Input: part model. Units: mm. Frame: model coordinates. A direction names the side the tool comes from. Coordinates: 2 decimals unless noted, no trailing zeros. Write each loop counter-clockwise with the first axis right and the second up, starting at its lowest first coordinate (ties: lowest second). Pieces come first, ordered by that corner, then holes. Notation, with made-up numbers: (0, 46.25) -> (11, 46.25) arc R21 cw to (11, 82.25) -> close; hole circle Ø3 at (58.25, 12). An arc over 180 degrees is marked (long way). Use one line per item in the form item = value. Start each with the question number.
(1) Cut plane D-D on x = -10.5. Return the cut outline in (y, z), plus the area to 3 significant figures.
(2) Cut plane C-C on y = -8. Return the cut outline in (x, z).
(3) Ray query, line 1 along Y through (x, z) = (0, -14); line 2 along Y through (x, z) = (0, 155); line 3 along X through (y, z) = (0, -15.25). Return the intervals inside material, ascending.
(4) Set-up query: faces 1 (the face through (0, 0, 8.44)), 2 (the face through (-4, -4, -35)). Return all of +Z, -Z, +X, -X, +Y, -Y with unobstructed straight access to the full face (end or side cutting, diameter ignored); none if empty.
(5) First-contact query: pin 1 (1 mm diameter, centred on x = 14, y = 0.5, fed in from +Z); pin 2 (8 mm diameter, centred on x = -7.5, z = 121, fed in from +Y); pin 3 (5 mm diameter, centred on x = -1.5, z = 101.5, fed in from -Y); pin 4 (1.7 mm diameter, centred on x = 4.5, y = 0, fed in from -Z). Flat tips, straight axial feed; report the tip coordinate or a pass-through.
(6) Cut plane B-B on z = 141. Return the cut outline in (x, y).
(7) Cut plane A-A on x = 0. Return the cut outline in (y, z).
(8) Pull-direction query (X, two-part tool) for faces 3 (the face through (3, 15, 208.44)), 4 (the face through (-1, 0, -10)); classes: released by +X, released by -X, zero draft, split by the parting line, or undercut.
```python
from build123d import *

# Parameters (mm, degrees)
SKETCH_1_R          = 20
EXTRUDE_1_DEPTH     = 208.44
EXTRUDE_START       = 35
SKETCH_3_R          = 20
EXTRUDE_2_DEPTH     = 35
CUT_EXTRUDE_1_DEPTH = 25
SKETCH_5_R          = 5
CUT_EXTRUDE_2_DEPTH = 10
SKETCH_6_R          = 15
CUT_EXTRUDE_3_DEPTH = 200


with BuildPart() as part:
    # 스케치1 → 보스-돌출1 (new body)
    with BuildSketch(Plane.XY):
        Circle(SKETCH_1_R)
    extrude(amount=EXTRUDE_1_DEPTH)

    # 스케치3 → 보스-돌출2 (add)
    with BuildSketch(Plane(origin=(0, 0, 0), x_dir=(-1, 0, 0), z_dir=(0, 0, -1)).offset(EXTRUDE_START)):
        Circle(SKETCH_3_R)
    extrude(amount=-EXTRUDE_2_DEPTH)

    # 스케치4 → 컷-돌출1 (cut)
    with BuildSketch(Plane(origin=(0, 0, -35), x_dir=(-1, 0, 0), z_dir=(0, 0, -1))):
        with BuildLine():
            Line((-3.515670801, 3.555286039), (-3.484261495, -3.586073317))
            ThreePointArc((-3.484261495, -3.586073317), (4.99995164, 0.021990913), (-3.515670801, 3.555286039))
        make_face()
    extrude(amount=-CUT_EXTRUDE_1_DEPTH, mode=Mode.SUBTRACT)

    # 스케치5 → 컷-돌출2 (cut)
    with BuildSketch(Plane(origin=(0, 0, -35), x_dir=(-1, 0, 0), z_dir=(0, 0, -1))):
        Circle(SKETCH_5_R)
    extrude(amount=-CUT_EXTRUDE_2_DEPTH, mode=Mode.SUBTRACT)

    # 스케치6 → 컷-돌출3 (cut)
    with BuildSketch(Plane.XY.offset(208.44)):
        Circle(SKETCH_6_R)
    extrude(amount=-CUT_EXTRUDE_3_DEPTH, mode=Mode.SUBTRACT)


solid = part.part
```
Values:
q1.outline = (-17.02, -35) -> (17.02, -35) -> (17.02, 208.44) -> (10.71, 208.44) -> (10.71, 8.44) -> (-10.71, 8.44) -> (-10.71, 208.44) -> (-17.02, 208.44) -> close
q1.area = 4,000 mm2
q2.outline = (-18.33, -35) -> (18.33, -35) -> (18.33, 208.44) -> (12.69, 208.44) -> (12.69, 8.44) -> (-12.69, 8.44) -> (-12.69, 208.44) -> (-18.33, 208.44) -> close
q3.line_1 = -20 to -5, 5 to 20
q3.line_2 = -20 to -15, 15 to 20
q3.line_3 = -20 to -5, 3.5 to 20
q4.face_1 = +Z
q4.face_2 = -Z, +X, -X, +Y, -Y
q5.pin_1 = 8.44
q5.pin_2 = 19.69
q5.pin_3 = -20
q5.pin_4 = -35
q6.outline = circle Ø40 at (0, 0); hole circle Ø30 at (0, 0)
q7.outline = (-20, -35) -> (-5, -35) -> (-5, -10) -> (5, -10) -> (5, -35) -> (20, -35) -> (20, 208.44) -> (15, 208.44) -> (15, 8.44) -> (-15, 8.44) -> (-15, 208.44) -> (-20, 208.44) -> close
q8.face_3 = zero draft
q8.face_4 = undercut
